Here's the drawing with two shaded views (mm, measured from the low corner). I have some questions. Give positions to 0.01 mm unless a question says otherwise; leave off trailing zeros. Loops run counter-clockwise (first coordinate to the right, second up) from the corner with the lowest first, then second, coordinate; pieces in that order, holes last. Notation, with made-up numbers: (47, -0.75) - (73, -0.75) arc R17 ccw to (73, 19.25) - close; hole circle Ø7 at (17.5, 34.5). An arc over 180 degrees is marked (long way). Use a Markdown table: item, result. Add a question column.
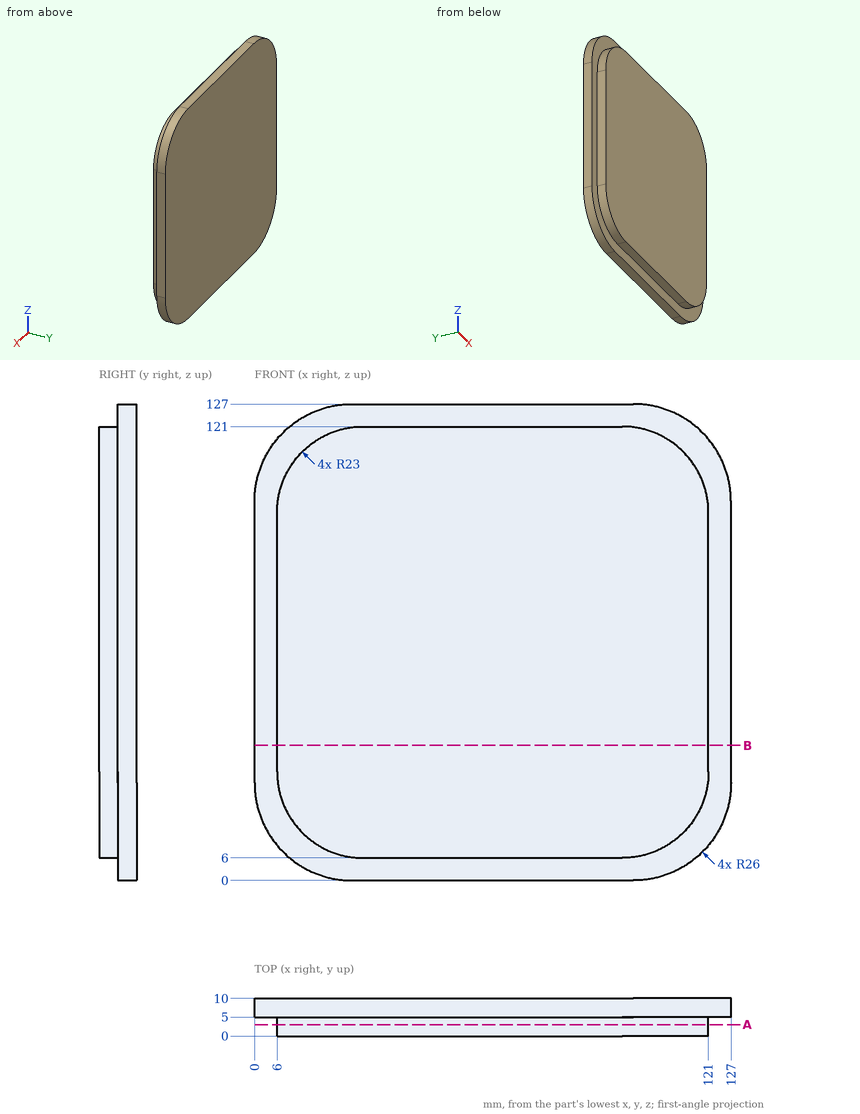
1. Please list where these lines run through material, in increasing order: line 1 along Y through (x, z) = (122.5, 14.5); line 2 along X through (y, z) = (1.5, 40). Write a range as [from, to].
2. Will these pins go through, and if not, where does the flat tip stop? P1, Ø4, axis at y = 2, z = 66.5, coming from the +X side; P2, Ø4, axis at x = 74, y = 2.5, coming from the +Z side; P3, Ø2, axis at y = 8.5, z = 20, coming from the -X side.
3. Suppose I cut it at B-B (z = 36). List the corners of the cut face in (x, y) for me.
4. Suppose I cut it at A-A (y = 3). List the corners of the cut face in (x, z) for me.
Results below:
| question | item | result |
|---|---|---|
| 1 | line 1 | [5, 10] |
| 1 | line 2 | [6, 121] |
| 2 | P1 | x = 121 |
| 2 | P2 | z = 121 |
| 2 | P3 | x = 0.49 |
| 3 | outline | (0, 5) - (6, 5) - (6, 0) - (121, 0) - (121, 5) - (127, 5) - (127, 10) - (0, 10) - close |
| 4 | outline | (6, 29) arc R23 ccw to (29, 6) - (98, 6) arc R23 ccw to (121, 29) - (121, 98) arc R23 ccw to (98, 121) - (29, 121) arc R23 ccw to (6, 98) - close |
